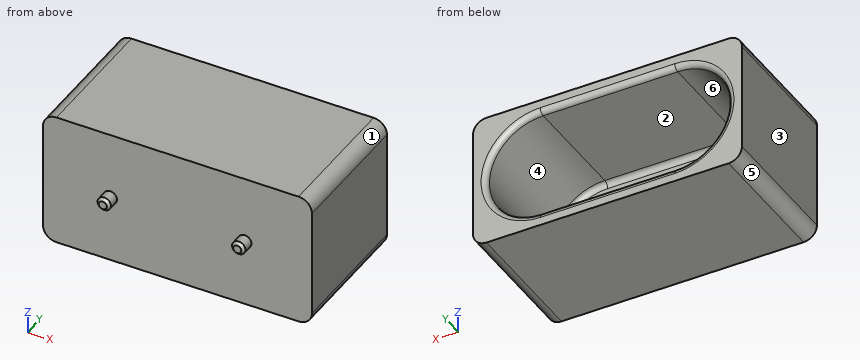
from build123d import *

# Parameters (mm, degrees)
SKETCH1_W           = 100
SKETCH1_H           = 50
BOSS_EXTRUDE1_DEPTH = 50
FILLET1_R           = 5
SKETCH2_R           = 2.5
BOSS_EXTRUDE2_DEPTH = 5
CHAMFER1_SIZE       = 1
CUT_EXTRUDE1_DEPTH  = 45
FILLET2_R           = 2


with BuildPart() as part:
    # Sketch1 → Boss-Extrude1 (new body)
    with BuildSketch(Plane(origin=(0, 0, 0), x_dir=(1, 0, 0), z_dir=(0, 1, 0))):
        Rectangle(SKETCH1_W, SKETCH1_H)
    extrude(amount=BOSS_EXTRUDE1_DEPTH)

    # Fillet1
    fillet1_edges = [part.edges().sort_by_distance(p)[0] for p in [
        (50, 25, 25),
        (-50, 25, 25),
        (-50, 25, -25),
        (50, 25, -25),
    ]]
    fillet(fillet1_edges, radius=FILLET1_R)

    # Sketch2 → Boss-Extrude2 (add)
    with BuildSketch(Plane.XZ):
        with Locations(Location((-25, 0, 0), (0, 0, 270))):
            Circle(SKETCH2_R)
        with Locations(Location((25, 0, 0), (0, 0, 270))):
            Circle(SKETCH2_R)
    extrude(amount=BOSS_EXTRUDE2_DEPTH)

    # Chamfer1
    chamfer1_edges = [part.edges().sort_by_distance(p)[0] for p in [
        (-25, -5, 2.5),
        (25, -5, 2.5),
    ]]
    chamfer(chamfer1_edges, length=CHAMFER1_SIZE)

    # Sketch3 → Cut-Extrude1 (cut)
    with BuildSketch(Plane(origin=(0, 50, 0), x_dir=(1, 0, 0), z_dir=(0, 1, 0))):
        with BuildLine():
            Line((-25, 20), (25, 20))
            ThreePointArc((25, 20), (45, 0), (25, -20))
            Line((25, -20), (-25, -20))
            ThreePointArc((-25, -20), (-45, 0), (-25, 20))
        make_face()
    extrude(amount=-CUT_EXTRUDE1_DEPTH, mode=Mode.SUBTRACT)

    # Fillet2
    fillet2_edges = [part.edges().sort_by_distance(p)[0] for p in [
        (-45, 50, 0),
        (0, 50, 20),
        (45, 50, 0),
        (0, 50, -20),
        (0, 5, 20),
        (45, 5, 0),
        (0, 5, -20),
        (-45, 5, 0),
    ]]
    fillet(fillet2_edges, radius=FILLET2_R)


solid = part.part
The model under review builds one solid part; all positions refer to its coordinate system, in mm. Face numbers are marked on the shaded views. A direction names the side the tool comes from. Give positions to 0.01 mm unless a question says otherwise; leave off trailing zeros. Order: outer loops, then holes, each group sorted by start corner. A loop starts at its lowest first (then second) coordinate and runs counter-clockwise, first axis right, second up. Notation, with made-up numbers: M 68,12.25 L 110,12.25 A33 ccw 110,45.25 Z; hole C 19,19.25 d9. An arc over 180 degrees is marked long. Use one line per item in the form item = value. Start each with the question number.
Item 1: To check wall thickness, follow line 1 along X through (y, z) = (37.5, 0); line 2 along Z through (x, y) = (-20, 47); line 3 along X through (y, z) = (19.5, 5). State the ranges of each line that lie inside material, in increasing order. Write a range as from..to.
Item 2: The part is to be moulded in two halves that separate along Z. For the marked faces 3, 4, 5 and 6, say which applies: pulls with the +Z half, pulls with the -Z half, needs draft (parallel to the pull), parting line crosses it, or undercut.
Item 3: We need section C-C on x = 2. Give the boundary of the cut face in (y, z), plus the area to 3 significant figures.
Item 4: We need section B-B on z = 0. Give the boundary of the cut face in (x, y).
Item 5: We need section A-A on y = 31.5. Give the boundary of the cut face in (x, z).
Item 6: Insertion check: pin 1 Ø6 at (x, z) = (-12.5, 10.5) entering from -Y. The pin has a flat end and moves straight along its axis. Give the tip position at first contact, or say it passes through.
Item 7: For the marked faces 1 and 2, list the 3-axis set-ups (+Z, -Z, +X, -X, +Y, -Y) from which the entire face can be reached by the end or side of a thin tool; tool diameter is ignored.
Completed:
q1.line_1 = -50..-45, 45..50
q1.line_2 = -25..-20, 20..25
q1.line_3 = -50..-44.36, 44.36..50
q2.face_3 = needs draft
q2.face_4 = undercut
q2.face_5 = pulls with the -Z half
q2.face_6 = undercut
q3.outline = M 0,-25 L 50,-25 L 50,-22 A2 ccw 48,-20 L 7,-20 A2 cw 5,-18 L 5,18 A2 cw 7,20 L 48,20 A2 ccw 50,22 L 50,25 L 0,25 Z
q3.area = 700 mm²
q4.outline = M -50,0 L -27.5,0 L -27.5,-4 L -26.5,-5 L -23.5,-5 L -22.5,-4 L -22.5,0 L 22.5,0 L 22.5,-4 L 23.5,-5 L 26.5,-5 L 27.5,-4 L 27.5,0 L 50,0 L 50,50 L 47,50 A2 ccw 45,48 L 45,7 A2 cw 43,5 L -43,5 A2 cw -45,7 L -45,48 A2 ccw -47,50 L -50,50 Z
q5.outline = M -50,-20 A5 ccw -45,-25 L 45,-25 A5 ccw 50,-20 L 50,20 A5 ccw 45,25 L -45,25 A5 ccw -50,20 Z; hole M -25,-20 L 25,-20 A20 ccw 25,20 L -25,20 A20 ccw Z
q6.pin_1 = 0
q7.face_1 = +Z, +X, +Y, -Y
q7.face_2 = +Y
